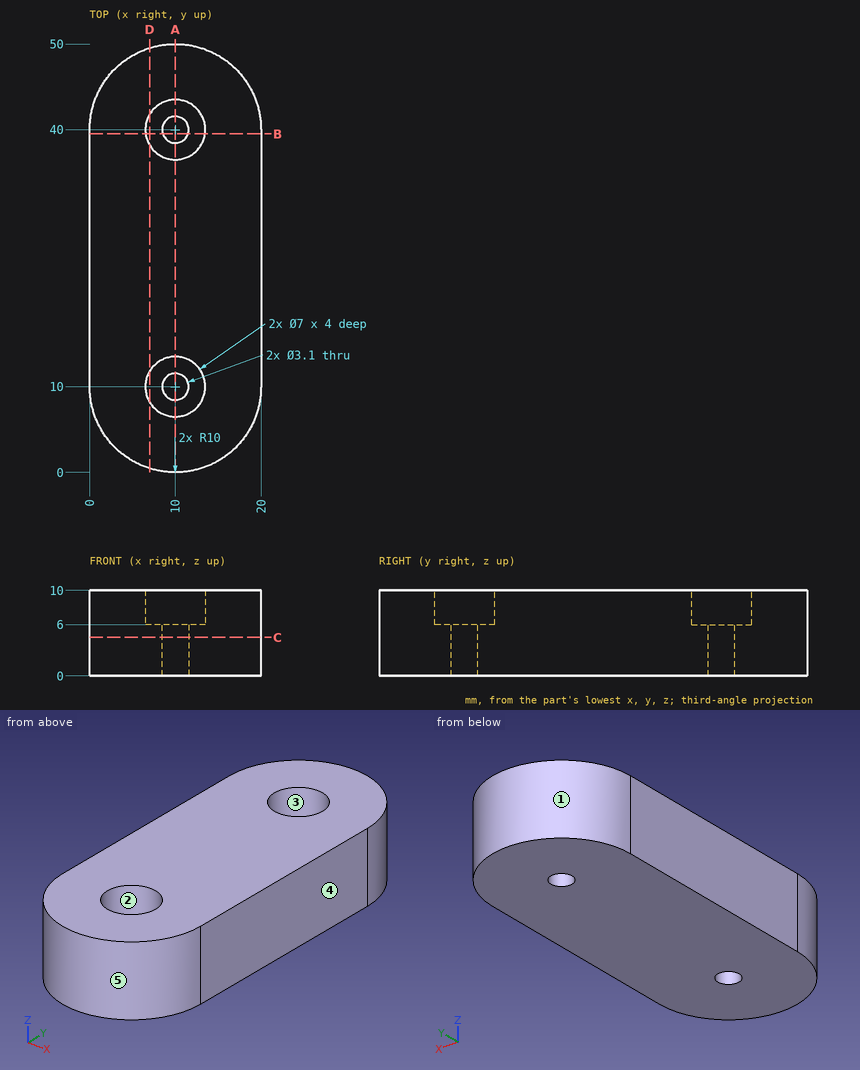
Design review of the part shown in the three views and the two pictorial views. Dimensions are in mm from the part's minimum x, y and z. A direction names the side the tool comes from. Round coordinates to 2 decimals unless told otherwise and drop trailing zeros. Write each loop counter-clockwise with the first axis right and the second up, starting at its lowest first coordinate (ties: lowest second). Pieces come first, ordered by that corner, then holes. Notation, with made-up numbers: M 31.25,12 L 49.25,12 A25 ccw 49.25,36 Z; hole C 59.25,26.5 d5. An arc over 180 degrees is marked long. One line per item, written item: value. Start each with the question number.
1. For the marked faces 1 and 2, list the 3-axis set-ups (+Z, -Z, +X, -X, +Y, -Y) from which the entire face can be reached by the end or side of a thin tool; tool diameter is ignored.
2. Take a section at A-A on x = 10. State the section outline as (y, z) points, then the cut area to 3 significant figures.
3. Take a section at B-B on y = 39.5. State the section outline as (x, z) points, then the cut area to 3 significant figures.
4. Take a section at C-C on z = 4.5. State the section outline as (x, y) points.
5. Draft analysis for pull direction Y (two halves, no side actions). For the marked faces 3, 4 and 5, state which applies: pulls with the +Y half, pulls with the -Y half, needs draft (parallel to the pull), parting line crosses it, or undercut.
6. Take a section at D-D on x = 7. State the section outline as (y, z) points.
7. To check wall thickness, follow probe 1 along Y at (x, z) = (10, 3.2); probe 2 along X at (y, z) = (40, 8.8); probe 3 along Y at (x, z) = (8.75, 4.5). State the ranges of each line that lie inside material, in increasing order. Write a range as from..to.
8. Clearance check with flat-ended pins moving along their axes: P1, Ø3.5, axis at x = 9.5, y = 8.5, coming from the +Z side; P2, Ø1.9, axis at x = 10, y = 40, coming from the +Z side; P3, Ø2, axis at x = 14, z = 5.5, coming from the +Y side. State where each tip first meets the part, or that it passes through.
Computed:
1. face 1: +Z, -Z, +Y
1. face 2: +Z
2. outline: M 0,0 L 8.45,0 L 8.45,6 L 6.5,6 L 6.5,10 L 0,10 Z; M 11.55,0 L 38.45,0 L 38.45,6 L 36.5,6 L 36.5,10 L 13.5,10 L 13.5,6 L 11.55,6 Z; M 41.55,0 L 50,0 L 50,10 L 43.5,10 L 43.5,6 L 41.55,6 Z
2. area: 407 mm²
3. outline: M 0,0 L 8.53,0 L 8.53,6 L 6.54,6 L 6.54,10 L 0,10 Z; M 11.47,0 L 20,0 L 20,10 L 13.46,10 L 13.46,6 L 11.47,6 Z
3. area: 155 mm²
4. outline: M 0,10 A10 ccw 20,10 L 20,40 A10 ccw 0,40 Z; hole C 10,10 d3.1; hole C 10,40 d3.1
5. face 3: undercut
5. face 4: needs draft
5. face 5: pulls with the -Y half
6. outline: M 0.46,0 L 49.54,0 L 49.54,10 L 41.8,10 L 41.8,6 L 38.2,6 L 38.2,10 L 11.8,10 L 11.8,6 L 8.2,6 L 8.2,10 L 0.46,10 Z
7. probe 1: y = 0..8.45, 11.55..38.45, 41.55..50
7. probe 2: x = 0..6.5, 13.5..20
7. probe 3: y = 0.08..9.08, 10.92..39.08, 40.92..49.92
8. P1: stops at z = 6
8. P2: passes through
8. P3: stops at y = 49.54
